```python
from build123d import *

# Parameters (mm, degrees)
BOSS_EXTRUDE1_DEPTH      = 19.57
BOSS_EXTRUDE1_DEPTH_BACK = 19.57
SKETCH1_R                = 25
SKETCH1_R_2              = 5
CUT_EXTRUDE1_START       = 19.57
SKETCH2_R                = 11
CUT_EXTRUDE1_DEPTH       = 7
CUT_EXTRUDE2_START       = -12.57
SKETCH3_R                = 11
CUT_EXTRUDE2_DEPTH       = 7
SKETCH4_R                = 15.875


with BuildPart() as part:
    # Sketch1 → Boss-Extrude1 (new, two sides: drawn at the far end of the back side and taken through both)
    with BuildSketch(Plane(origin=(0, 0, 0), x_dir=(0, 0, -1), z_dir=(1, 0, 0)).offset(-BOSS_EXTRUDE1_DEPTH_BACK)):
        Circle(SKETCH1_R)
        Circle(SKETCH1_R_2, mode=Mode.SUBTRACT)
    extrude(amount=BOSS_EXTRUDE1_DEPTH + BOSS_EXTRUDE1_DEPTH_BACK)

    # Sketch2 → Cut-Extrude1 (cut)
    with BuildSketch(Plane(origin=(0, 0, 0), x_dir=(0, 0, -1), z_dir=(1, 0, 0)).offset(CUT_EXTRUDE1_START)):
        Circle(SKETCH2_R)
    extrude(amount=-CUT_EXTRUDE1_DEPTH, mode=Mode.SUBTRACT)

    # Sketch3 → Cut-Extrude2 (cut)
    with BuildSketch(Plane(origin=(0, 0, 0), x_dir=(0, 0, -1), z_dir=(1, 0, 0)).offset(CUT_EXTRUDE2_START)):
        Circle(SKETCH3_R)
    extrude(amount=-CUT_EXTRUDE2_DEPTH, mode=Mode.SUBTRACT)

    # Sketch4 → Cut-Revolve1 (revolve, cut)
    with BuildSketch(Plane.XY, mode=Mode.PRIVATE) as cut_revolve1_sk:
        with Locations((0, 30.875)):
            Circle(SKETCH4_R)
    revolve(cut_revolve1_sk.sketch.rotate(Axis((0, 0, 0), (1, 0, 0)), 270), axis=Axis((0, 0, 0), (1, 0, 0)), mode=Mode.SUBTRACT)


solid = part.part
```
Here's how the part is built. I have some questions about the finished solid (model axes, mm). A direction names the side the tool comes from. Coordinates: 2 decimals unless noted, no trailing zeros. Loops run counter-clockwise (first coordinate to the right, second up) from the corner with the lowest first, then second, coordinate; pieces in that order, holes last. Notation, with made-up numbers: (85.5, 45.5) - (112.5, 45.5) arc R31 cw to (112.5, 81.5) - close; hole circle Ø8 at (23.25, 50.25). An arc over 180 degrees is marked (long way). Return JSON: item names as keys, results as strings. Group by question number.
Item 1: On a 3-axis mill with a long thin cutter (end or side, diameter ignored), from which of +Z, -Z, +X, -X, +Y, -Y can I reach the whole of each face in a straight line? I mean faces 4 (the face through (-0.18, -4.88, 1.08)), 5 (the face through (16.12, -10.74, 2.38)), 6 (the face through (-16.02, -10.74, 2.38)). Say none if no direction works.
Item 2: Will these pins go through, and if not, where does the flat tip stop? P1, Ø17.5, axis at y = 1, z = 1.5, coming from the +X side; P2, Ø8, axis at x = 7, y = -17.5, coming from the +Z side; P3, Ø2, axis at x = 2, z = -8.5, coming from the -Y side.
Item 3: We'd pull the mould along Y, two halves only. Please class faces 1 (the face through (-17.193, 7.509, -23.846)), 2 (the face through (12.57, -5, -2)), 3 (the face through (-19.57, -11, -5)): +Y half, -Y half, draft (parallel to the pull), parting line (faces both ways), or undercut.
Item 4: If we section it at C-C on x = -4.5: Write out the boundary of the cut face in (y, z).
Item 5: If we section it at A-A on y = 0: Write out the boundary of the cut face in (x, z) (3 decimals).
Item 6: I need wall thicknesses on line 1 (X direction, y = 6.5, z = -8); line 2 (X direction, y = -18, z = 12); line 3 (X direction, y = -11, z = -11.5). Which ranges of each line are inside material? Lowest first, please. Write a range as from..to.
Calculated:
{
 "1": {"face 4": "+X, -X", "face 5": "+X", "face 6": "-X"},
 "2": {"P1": "stops at x = 12.57", "P2": "stops at z = 11.12", "P3": "stops at y = -13.16"},
 "3": {"face 1": "parting line", "face 2": "undercut", "face 3": "draft"},
 "4": {"outline": "circle Ø31.3 at (0, 0); hole circle Ø10 at (0, 0)"},
 "5": {"outline": "(-19.57, -25) - (-14.748, -25) arc R15.875 cw to (14.748, -25) - (19.57, -25) - (19.57, -11) - (12.57, -11) - (12.57, -5) - (-12.57, -5) - (-12.57, -11) - (-19.57, -11) - close; (-19.57, 11) - (-12.57, 11) - (-12.57, 5) - (12.57, 5) - (12.57, 11) - (19.57, 11) - (19.57, 25) - (14.748, 25) arc R15.875 cw to (-14.748, 25) - (-19.57, 25) - close"},
 "6": {"line 1": "x = -12.57..12.57", "line 2": "x = -19.57..-12.91, 12.91..19.57", "line 3": "x = -19.57..-5.31, 5.31..19.57"}
}
